from build123d import *

# Parameters (mm, degrees)
SKETCH_1_W             = 250
SKETCH_1_H             = 250
SM_BASE_FLANGE_1_DEPTH = 8
CUT_EXTRUDE_1_DEPTH    = 10
CUT_EXTRUDE_2_DEPTH    = 10


# Sheet-metal steps are written as plain solids
with BuildPart() as part:
    # Sketch 1 → Базовая кромка1 (new body)
    with BuildSketch(Plane.XY):
        with Locations((125, -125)):
            Rectangle(SKETCH_1_W, SKETCH_1_H)
    extrude(amount=-SM_BASE_FLANGE_1_DEPTH)

    # Sketch 2 → Вырез-Вытянуть1 (cut)
    with BuildSketch(Plane.XY):
        Polygon((58.022064768, 0), (0, -68.8), (0, 0), align=None)
        Polygon((250, 0), (191.977935232, 0), (250, -68.8), align=None)
        Polygon((191.977935232, -250), (250, -181.2), (250, -250), align=None)
        Polygon((0, -250), (58.022064768, -250), (0, -181.2), align=None)
    extrude(amount=-CUT_EXTRUDE_1_DEPTH, mode=Mode.SUBTRACT)

    # Эскиз3 → Вырез-Вытянуть2 (cut)
    with BuildSketch(Plane(origin=(0, 0, -8), x_dir=(-1, 0, 0), z_dir=(0, 0, -1))):
        with BuildLine():
            Line((-69.557250856, -29.753839407), (-59.886906728, -41.220506074))
            ThreePointArc((-59.886906728, -41.220506074), (-60.725190579, -51.084444444), (-70.58912895, -50.246160593))
            Line((-70.58912895, -50.246160593), (-80.259473078, -38.779493926))
            ThreePointArc((-80.259473078, -38.779493926), (-79.421189227, -28.915555556), (-69.557250856, -29.753839407))
        make_face()
        with BuildLine():
            Line((-43.769666514, -60.331617185), (-34.099322386, -71.798283851))
            ThreePointArc((-34.099322386, -71.798283851), (-34.937606238, -81.662222222), (-44.801544609, -80.823938371))
            Line((-44.801544609, -80.823938371), (-54.471888737, -69.357271704))
            ThreePointArc((-54.471888737, -69.357271704), (-53.633604885, -59.493333333), (-43.769666514, -60.331617185))
        make_face()
        with BuildLine():
            Line((-180.442749144, -29.753839407), (-190.113093272, -41.220506074))
            ThreePointArc((-190.113093272, -41.220506074), (-189.274809421, -51.084444444), (-179.41087105, -50.246160593))
            Line((-179.41087105, -50.246160593), (-169.740526922, -38.779493926))
            ThreePointArc((-169.740526922, -38.779493926), (-170.578810773, -28.915555556), (-180.442749144, -29.753839407))
        make_face()
        with BuildLine():
            Line((-206.230333486, -60.331617185), (-215.900677614, -71.798283851))
            ThreePointArc((-215.900677614, -71.798283851), (-215.062393762, -81.662222222), (-205.198455391, -80.823938371))
            Line((-205.198455391, -80.823938371), (-195.528111263, -69.357271704))
            ThreePointArc((-195.528111263, -69.357271704), (-196.366395115, -59.493333333), (-206.230333486, -60.331617185))
        make_face()
        with BuildLine():
            Line((-69.557250856, -220.246160593), (-59.886906728, -208.779493926))
            ThreePointArc((-59.886906728, -208.779493926), (-60.725190579, -198.915555556), (-70.58912895, -199.753839407))
            Line((-70.58912895, -199.753839407), (-80.259473078, -211.220506074))
            ThreePointArc((-80.259473078, -211.220506074), (-79.421189227, -221.084444444), (-69.557250856, -220.246160593))
        make_face()
        with BuildLine():
            Line((-43.769666514, -189.668382815), (-34.099322386, -178.201716149))
            ThreePointArc((-34.099322386, -178.201716149), (-34.937606238, -168.337777778), (-44.801544609, -169.176061629))
            Line((-44.801544609, -169.176061629), (-54.471888737, -180.642728296))
            ThreePointArc((-54.471888737, -180.642728296), (-53.633604885, -190.506666667), (-43.769666514, -189.668382815))
        make_face()
        with BuildLine():
            Line((-180.442749144, -220.246160593), (-190.113093272, -208.779493926))
            ThreePointArc((-190.113093272, -208.779493926), (-189.274809421, -198.915555556), (-179.41087105, -199.753839407))
            Line((-179.41087105, -199.753839407), (-169.740526922, -211.220506074))
            ThreePointArc((-169.740526922, -211.220506074), (-170.578810773, -221.084444444), (-180.442749144, -220.246160593))
        make_face()
        with BuildLine():
            Line((-206.230333486, -189.668382815), (-215.900677614, -178.201716149))
            ThreePointArc((-215.900677614, -178.201716149), (-215.062393762, -168.337777778), (-205.198455391, -169.176061629))
            Line((-205.198455391, -169.176061629), (-195.528111263, -180.642728296))
            ThreePointArc((-195.528111263, -180.642728296), (-196.366395115, -190.506666667), (-206.230333486, -189.668382815))
        make_face()
    extrude(amount=-CUT_EXTRUDE_2_DEPTH, mode=Mode.SUBTRACT)


solid = part.part
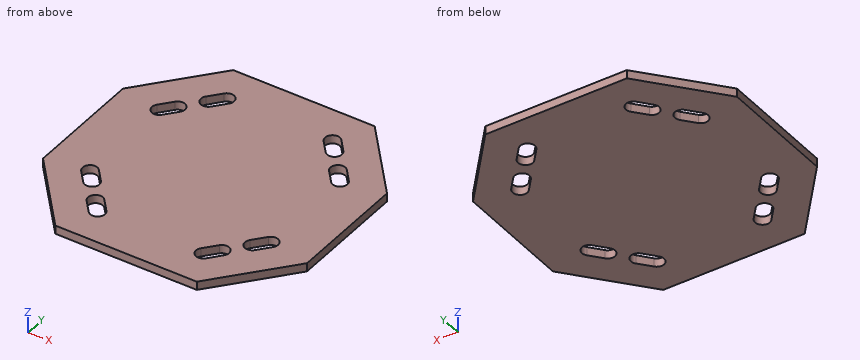
Work out the finished part from the listing and answer in its coordinate system (mm). Round coordinates to 2 decimals unless told otherwise and drop trailing zeros. Loops run counter-clockwise (first coordinate to the right, second up) from the corner with the lowest first, then second, coordinate; pieces in that order, holes last. Notation, with made-up numbers: (-27.75, 86) - (-8.75, 86) arc R18 cw to (-8.75, 93) - close; hole circle Ø3 at (39, 57.5). An arc over 180 degrees is marked (long way). One line per item, written item: value.
Q1. Each of these flat-tipped pins is pushed along its axis until it touches: pin 1 Ø5 at (x, y) = (58.5, -53.5) entering from +Z; pin 2 Ø4 at (y, z) = (-33, -6) entering from +X (3 decimals). Where does it stop, or does it pass through?
Check values:
pin 1: z = 0
pin 2: x = 221.495
Q2. Straight lines are drawn through the part: probe 1 along Y at (x, z) = (54.5, -0.25); probe 2 along Y at (x, z) = (183, -5.5); probe 3 along X at (y, z) = (-51.5, -1.5). For each, find the intervals that lie inside material, in ascending order.
Check values:
probe 1: -245.82 to -189.63, -180.68 to -69.32, -60.37 to -4.18
probe 2: -250 to -217.21, -197.49 to -52.51, -32.79 to 0
probe 3: 14.59 to 61.27, 69.21 to 180.79, 188.73 to 235.41
Q3. Find section A-A on x = 38. Give the vertices of the cut face in (y, z), and give its area (3 significant figures).
Check values:
outline: (-226.26, -8) - (-182.83, -8) - (-182.83, 0) - (-226.26, 0) - close; (-166.84, -8) - (-83.16, -8) - (-83.16, 0) - (-166.84, 0) - close; (-67.17, -8) - (-23.74, -8) - (-23.74, 0) - (-67.17, 0) - close
area: 1,360 mm2
Q4. Find section B-B on z = -2.5. State how many separate pieces and enclosed holes the cut face has, and give its area (3 significant figures).
Check values:
separate pieces: 1
enclosed holes: 8
area: 51,600 mm2
